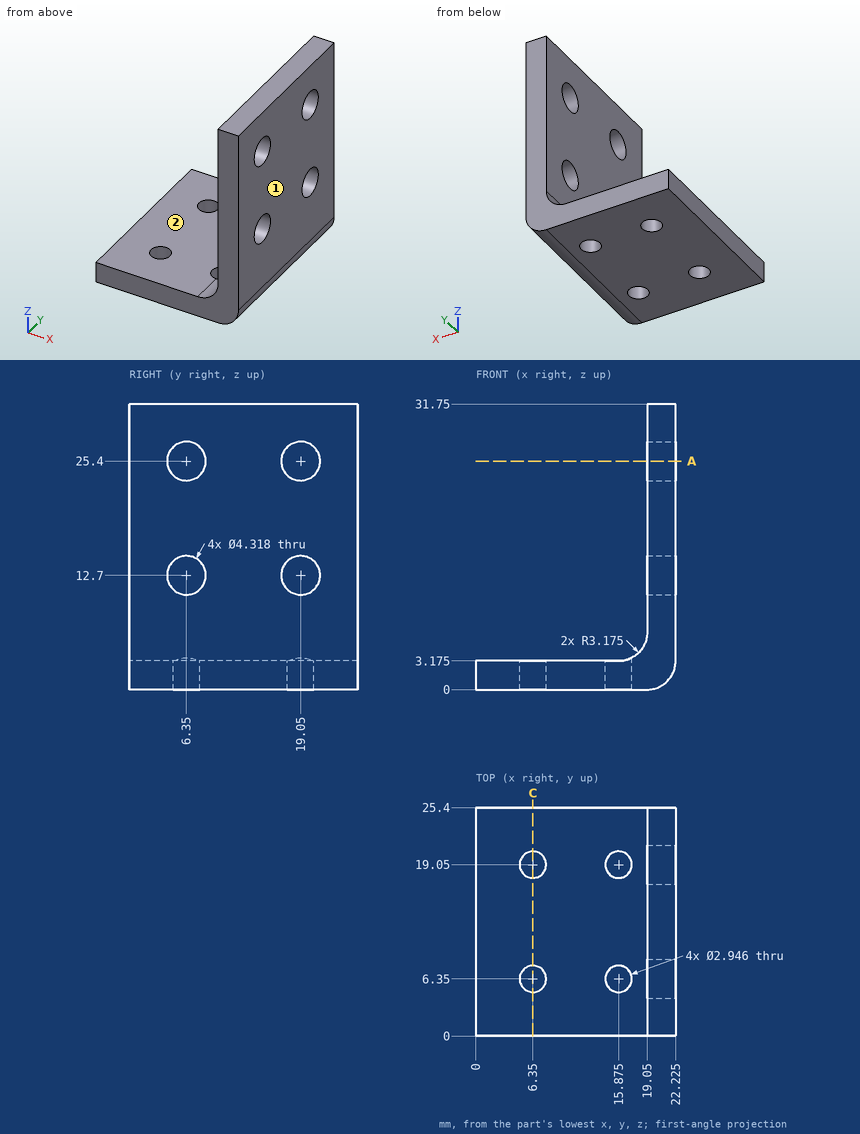
Geometry: see drawing. Coordinates: mm, zero at the bounding-box minimum. A direction names the side the tool comes from. Give positions to 0.01 mm unless a question says otherwise; leave off trailing zeros. Loops run counter-clockwise (first coordinate to the right, second up) from the corner with the lowest first, then second, coordinate; pieces in that order, holes last. Notation, with made-up numbers: (12.25, 8) -> (43.25, 8) arc R18 ccw to (43.25, 37) -> close; hole circle Ø1 at (57, 79). An arc over 180 degrees is marked (long way). Put each result on its own line as item: value.
1. Cut plane A-A (z = 25.4). Count the separate pieces of the cut face and the enclosed holes in it.
Taken from the geometry:
separate pieces: 3
enclosed holes: 0
2. Ray query, line 1 along Z through (x, y) = (19.95, 6.35); line 2 along Z through (x, y) = (16, 16.25); line 3 along X through (y, z) = (6.25, 5.5) (1 decimal). Return the intervals inside material, ascending. Write a range as [from, to].
Taken from the geometry:
line 1: z = [0.13, 10.54], [14.86, 23.24], [27.56, 31.75]
line 2: z = [0, 3.18]
line 3: x = [18.9, 22.2]
3. Set-up query: the marked faces 1 and 2. Return all of +Z, -Z, +X, -X, +Y, -Y with unobstructed straight access to the full face (end or side cutting, diameter ignored); none if empty.
Taken from the geometry:
face 1: +Z, -Z, +X, +Y, -Y
face 2: +Z, -X, +Y, -Y
4. Cut plane C-C (x = 6.35). Return the cut outline in (y, z) (1 decimal).
Taken from the geometry:
outline: (0, 0) -> (4.9, 0) -> (4.9, 3.2) -> (0, 3.2) -> close; (7.8, 0) -> (17.6, 0) -> (17.6, 3.2) -> (7.8, 3.2) -> close; (20.5, 0) -> (25.4, 0) -> (25.4, 3.2) -> (20.5, 3.2) -> close
5. Pin query (flat end, axial travel): P1, Ø5.5, axis at y = 19.05, z = 25.4, coming from the -X side; P2, Ø4.5, axis at x = 6.35, y = 6.35, coming from the +Z side (3 decimals); P3, Ø4.5, axis at x = 15.875, y = 6.35, coming from the +Z side. Return the tip coordinate at first contact, or that it passes through.
Taken from the geometry:
P1: stops at x = 19.05
P2: stops at z = 3.175
P3: stops at z = 4.11
